Geometry: final body of the model. Coordinates: model frame, mm. A direction names the side the tool comes from. Give positions to 0.01 mm unless a question says otherwise; leave off trailing zeros. Order: outer loops, then holes, each group sorted by start corner. A loop starts at its lowest first (then second) coordinate and runs counter-clockwise, first axis right, second up. Notation, with made-up numbers: (63.25, 32) - (104.25, 32) arc R16 cw to (104.25, 42) - close; hole circle Ø6 at (-9, 57). An arc over 180 degrees is marked (long way). Write item = value, one per line. Start each with the question number.
from build123d import *

# Parameters (mm, degrees)
ESQUISSE1_R        = 2
ESQUISSE1_W        = 5
ESQUISSE1_H        = 5
BOSS_EXTRU_1_DEPTH = 5


with BuildPart() as part:
    # Esquisse1 → Boss.-Extru.1 (new body)
    with BuildSketch(Plane.XY):
        Polygon((-10, 100), (-15, 100), (-15, 0), (-5, -20), (5, -20), (15, 0), (15, 100), (10, 100), (10, 105), (5, 105), (5, 100), (2, 100), (2, 97), (3.5, 97), (3.5, 94), (2, 94), (2, 90), (-2, 90), (-2, 94), (-3.5, 94), (-3.5, 97), (-2, 97), (-2, 100), (-5, 100), (-5, 105), (-10, 105), align=None)
        with Locations((0, 40)):
            Circle(ESQUISSE1_R, mode=Mode.SUBTRACT)
        with Locations((0, 20)):
            Circle(ESQUISSE1_R, mode=Mode.SUBTRACT)
        Circle(ESQUISSE1_R, mode=Mode.SUBTRACT)
        with Locations((0, 60)):
            Circle(ESQUISSE1_R, mode=Mode.SUBTRACT)
        with Locations((0, 80)):
            Circle(ESQUISSE1_R, mode=Mode.SUBTRACT)
        with Locations((-7.5, 40)):
            Rectangle(ESQUISSE1_W, ESQUISSE1_H, mode=Mode.SUBTRACT)
        with Locations((7.5, 40)):
            Rectangle(ESQUISSE1_W, ESQUISSE1_H, mode=Mode.SUBTRACT)
        with Locations((-7.5, 20)):
            Rectangle(ESQUISSE1_W, ESQUISSE1_H, mode=Mode.SUBTRACT)
        with Locations((7.5, 20)):
            Rectangle(ESQUISSE1_W, ESQUISSE1_H, mode=Mode.SUBTRACT)
        with Locations((-7.5, 0)):
            Rectangle(ESQUISSE1_W, ESQUISSE1_H, mode=Mode.SUBTRACT)
        with Locations((7.5, 0)):
            Rectangle(ESQUISSE1_W, ESQUISSE1_H, mode=Mode.SUBTRACT)
        with Locations((-7.5, 60)):
            Rectangle(ESQUISSE1_W, ESQUISSE1_H, mode=Mode.SUBTRACT)
        with Locations((7.5, 60)):
            Rectangle(ESQUISSE1_W, ESQUISSE1_H, mode=Mode.SUBTRACT)
        with Locations((-7.5, 80)):
            Rectangle(ESQUISSE1_W, ESQUISSE1_H, mode=Mode.SUBTRACT)
        with Locations((7.5, 80)):
            Rectangle(ESQUISSE1_W, ESQUISSE1_H, mode=Mode.SUBTRACT)
    extrude(amount=BOSS_EXTRU_1_DEPTH)


solid = part.part
Q1. Section B-B, the plane x = -8.25. Return the cut outline in (y, z).
Q2. Section A-A, the plane y = 60. Return the cut outline in (x, z), then the cut area to 3 significant figures.
Q3. Set-up query: faces 1 (the flat face through (-3, 100, 2)), 2 (the flat face through (10, 20, 2)), 3 (the flat face through (-10, 103, 2)), 4 (the flat face through (13, 100, 2)). Return all of +Z, -Z, +X, -X, +Y, -Y with unobstructed straight access to the full face (end or side cutting, diameter ignored); none if empty.
Q4. Pull-direction query (Y, two-part tool) for faces 5 (the flat face through (0, 43, 5)), 6 (the flat face through (10, -10, 2)), 7 (the cylindrical face through (0, -2, 2)); classes: +Y half, -Y half, draft (parallel to the pull), parting line (faces both ways), or undercut.
Q5. Contact query for flat-ended pins moving along their axis: pin 1 (1.5 mm diameter, centred on y = 101.5, z = 3, fed in from +X); pin 2 (2.5 mm diameter, centred on x = 8.5, z = 3, fed in from -Y). Output: stop coordinate, or through.
Q6. Section C-C, the plane z = 2.6. Count the separate pieces of the cut face and the enclosed holes in it, then the cut area to 3 significant figures.
Q7. Section D-D, the plane y = -8.5. Return the cut outline in (x, z), then the cut area to 4 significant figures.
Q8. Material intervals for line 1 along Y through (x, z) = (0, 2.15); line 2 along Y through (x, z) = (-2.75, 2.75); line 3 along Y through (x, z) = (9, 3.25), sorted ascending. Write a range as from..to.
The answers:
q1.outline = (-13.5, 0) - (-2.5, 0) - (-2.5, 5) - (-13.5, 5) - close; (2.5, 0) - (17.5, 0) - (17.5, 5) - (2.5, 5) - close; (22.5, 0) - (37.5, 0) - (37.5, 5) - (22.5, 5) - close; (42.5, 0) - (57.5, 0) - (57.5, 5) - (42.5, 5) - close; (62.5, 0) - (77.5, 0) - (77.5, 5) - (62.5, 5) - close; (82.5, 0) - (105, 0) - (105, 5) - (82.5, 5) - close
q2.outline = (-15, 0) - (-10, 0) - (-10, 5) - (-15, 5) - close; (-5, 0) - (-2, 0) - (-2, 5) - (-5, 5) - close; (2, 0) - (5, 0) - (5, 5) - (2, 5) - close; (10, 0) - (15, 0) - (15, 5) - (10, 5) - close
q2.area = 80.0 mm²
q3.face_1 = +Z, -Z, +Y
q3.face_2 = +Z, -Z
q3.face_3 = +Z, -Z, -X, +Y
q3.face_4 = +Z, -Z, +X, +Y
q4.face_5 = draft
q4.face_6 = -Y half
q4.face_7 = undercut
q5.pin_1 = 10
q5.pin_2 = -15.5
q6.separate_pieces = 1
q6.enclosed_holes = 15
q6.area = 3,090 mm²
q7.outline = (-10.75, 0) - (10.75, 0) - (10.75, 5) - (-10.75, 5) - close
q7.area = 107.5 mm²
q8.line_1 = -20..-2, 2..18, 22..38, 42..58, 62..78, 82..90
q8.line_2 = -20..94, 97..100
q8.line_3 = -12..-2.5, 2.5..17.5, 22.5..37.5, 42.5..57.5, 62.5..77.5, 82.5..105
